Read the model definition and answer for the solid it produces. Units are mm, in the model's axes. Coordinates: 2 decimals unless noted, no trailing zeros. Write each loop counter-clockwise with the first axis right and the second up, starting at its lowest first coordinate (ties: lowest second). Pieces come first, ordered by that corner, then holes. Notation, with made-up numbers: (15, 70.5) -> (59, 70.5) arc R13 cw to (59, 76.5) -> close; hole circle Ø3 at (-37, 19). An arc over 180 degrees is marked (long way). Answer as a JSON object with one key per item and string values. Group by question number.
(1) Straight lines are drawn through the part: L1, parallel to X at y = -155.25, z = 254; L2, parallel to Y at x = -642, z = 281.5; L3, parallel to X at y = -164.5, z = 301. For each, find the intervals that lie inside material, in ascending order.
(2) Find section A-A (y = -161). Give the vertices of the cut face in (x, z), then the cut area to 3 significant figures.
(3) Flat-ended cylindrical pins translate along their axes: P1, Ø3, axis at x = -629.5, z = 248.5, coming from the +Y side; P2, Ø12, axis at x = -630.5, y = -153.5, coming from the -Z side; P3, Ø6, axis at x = -632, z = 251.5, coming from the +Y side; P4, Ø1, axis at y = -164.5, z = 282.5, coming from the +X side. Find the tip coordinate at first contact, or state that the pin passes through.
(4) Find section B-B (x = -636). Give the vertices of the cut face in (y, z).
(5) For a pull along X with two mould halves and no side action, classify faces 1 (the face through (-630.026, -156.229, 285.831)), 2 (the face through (-630.94, -157.996, 285.623)), 3 (the face through (-632.54, -155.94, 284.73)) as +X half, -X half, draft (parallel to the pull), parting line (faces both ways), or undercut.
Autodesk Inventor part; units mm, degrees
ref_plane "YZ Plane" through (0, 0, 0) normal (1, 0, 0) x (0, 1, 0)
ref_plane "XZ Plane" through (0, 0, 0) normal (0, 1, 0) x (-1, 0, 0)
ref_plane "XY Plane" through (0, 0, 0) normal (0, 0, 1) x (1, 0, 0)
ref_plane "Work Plane1" through (-728.8112, -105.3847, 288.112) normal (-0.4570507, -0.8833415, -0.1039826) x (0.88913, -0.4568478, -0.0271666)
sketch "Sketch1" plane through (-728.8112, -105.3847, 288.112) normal (-0.4570507, -0.8833415, -0.1039826) x (0.88913, -0.4568478, -0.0271666)
  line L0 (-49.7406, -45) -> (-49.7406, -53)
  line L1 (-49.7406, -53) -> (123, -53)
  line L2 (123, -53) -> (123, 53)
  line L3 (123, 53) -> (-49.7406, 53)
  line L4 (-49.7406, 53) -> (-49.7406, 45)
  line L5 (-49.7406, 45) -> (-91.8594, 45)
  line L6 (-91.8594, 45) -> (-91.8594, 53)
  line L7 (-91.8594, 53) -> (-123, 53)
  line L8 (-123, 53) -> (-123, -53)
  line L9 (-123, -53) -> (-91.8594, -53)
  line L10 (-91.8594, -53) -> (-91.8594, -45)
  line L11 (-91.8594, -45) -> (-49.7406, -45)
  line L12 (-95.4, -15.0028) -> (-111.4, -15.0028)
  line L13 (-111.4, -15.0028) -> (-111.4, 13.9972)
  line L14 (-111.4, 13.9972) -> (-95.4, 13.9972)
  line L15 (-95.4, 13.9972) -> (-95.4, -15.0028)
  line L16 (123, 53) -> (93, 53)
  line L17 (93, 53) -> (93, -53)
  line L18 (93, -53) -> (123, -53)
  line L19 (123, -53) -> (123, 53)
  point P0 (607.6902, -314.6271)
  dimension "d0" = 30
extrude "Extrusion1" add sketch "Sketch1" along normal blind 2 contours L17 L3 L2 L1
sketch "Sketch4" plane through (-729.7253, -107.1513, 287.9041) normal (-0.4570507, -0.8833415, -0.1039826) x (0.88913, -0.4568478, -0.0271666)
  circle A0 centre (108, 0) radius 0.85
  point P0 (607.6902, -314.6271)
extrude "Extrusion4" cut sketch "Sketch4" against normal up to next
thread "Thread1"
properties part number "Fram"
Results below:
{
 "1": {"L1": "x = -629.05 to -624.68", "L2": "y = -151.79 to -149.52", "L3": "x = -621.87 to -620.45"},
 "2": {"outline": "(-636.99, 337.73) -> (-619.84, 262.34) -> (-619.32, 279.3) -> (-632.63, 337.83) -> close", "area": "293 mm2"},
 "3": {"P1": "stops at y = -151.31", "P2": "stops at z = 232.04", "P3": "stops at y = -149.57", "P4": "passes through"},
 "4": {"outline": "(-161.51, 337.7) -> (-149.11, 232.39) -> (-146.87, 232.62) -> (-159.27, 337.93) -> close"},
 "5": {"face 1": "+X half", "face 2": "-X half", "face 3": "undercut"}
}
